```python
from build123d import *

# Parameters (mm, degrees)
SKETCH1_R           = 43.5
BOSS_EXTRUDE1_DEPTH = 122
EXTRUDE_THIN1_START = 0.5
SKETCH1_4_R         = 30.5
SKETCH1_4_R_2       = 30
EXTRUDE_THIN1_DEPTH = 115.5
BOSS_EXTRUDE2_START = 0.8
SKETCH1_5_R         = 42.5
SKETCH1_5_R_2       = 30
BOSS_EXTRUDE2_DEPTH = 115
BOSS_EXTRUDE3_START = 0.3
SKETCH1_6_R         = 43.5
SKETCH1_6_R_2       = 42.5
BOSS_EXTRUDE3_DEPTH = 117
BOSS_EXTRUDE4_START = 1
BOSS_EXTRUDE4_DEPTH = 1
FILLET1_R           = 0.5
SKETCH4_R           = 5.35
CUT_EXTRUDE3_DEPTH  = 180.543866506
CHAMFER1_SIZE       = 1


with BuildPart() as part:
    # Sketch1 → Boss-Extrude1 (new body)
    with BuildSketch(Plane(origin=(0, 0, 0), x_dir=(0, 0, -1), z_dir=(1, 0, 0))):
        Polygon((-66, -28), (-64.5, -26.5), (-64.5, 36), (-43.5, 36), (-22.5, 56), (22.5, 56), (43.5, 36), (64.5, 36), (64.5, -26.5), (66, -28), (66, -58), (26, -58), (24.5, -56.5), (-24.5, -56.5), (-26, -58), (-66, -58), align=None)
        with Locations(Location((0, 0, 0), (0, 0, 180))):
            Circle(SKETCH1_R, mode=Mode.SUBTRACT)
    extrude(amount=BOSS_EXTRUDE1_DEPTH)



with BuildPart() as body_2:
    # Sketch1_4 → Extrude-Thin1 (new body)
    with BuildSketch(Plane(origin=(0, 0, 0), x_dir=(0, 0, -1), z_dir=(1, 0, 0)).offset(EXTRUDE_THIN1_START)):
        Circle(SKETCH1_4_R)
        Circle(SKETCH1_4_R_2, mode=Mode.SUBTRACT)
    extrude(amount=EXTRUDE_THIN1_DEPTH)

    # Sketch1_5 → Boss-Extrude2 (add)
    with BuildSketch(Plane(origin=(0, 0, 0), x_dir=(0, 0, -1), z_dir=(1, 0, 0)).offset(BOSS_EXTRUDE2_START)):
        Circle(SKETCH1_5_R)
        Circle(SKETCH1_5_R_2, mode=Mode.SUBTRACT)
    extrude(amount=BOSS_EXTRUDE2_DEPTH)


with BuildPart() as part_1:
    add(part.part)

    add(body_2.part)  # Boss-Extrude3 merges body 2
    # Sketch1_6 → Boss-Extrude3 (add)
    with BuildSketch(Plane(origin=(0, 0, 0), x_dir=(0, 0, -1), z_dir=(1, 0, 0)).offset(BOSS_EXTRUDE3_START)):
        with Locations(Location((0, 0, 0), (0, 0, 180))):
            Circle(SKETCH1_6_R)
        Circle(SKETCH1_6_R_2, mode=Mode.SUBTRACT)
    extrude(amount=BOSS_EXTRUDE3_DEPTH)

    # Sketch3 → Boss-Extrude4 (add)
    with BuildSketch(Plane(origin=(117.3, 0, 0), x_dir=(0, 0, -1), z_dir=(1, 0, 0)).offset(BOSS_EXTRUDE4_START)):
        with BuildLine():
            Line((-1.000623377, -42.488218989), (-1.024167456, -43.487941789))
            ThreePointArc((-1.024167456, -43.487941789), (0, 43.5), (1.024167456, -43.487941789))
            Line((1.024167456, -43.487941789), (1.000623377, -42.488218989))
            ThreePointArc((1.000623377, -42.488218989), (1.691854541, -41.50157584), (2.830286494, -41.895578267))
            ThreePointArc((2.830286494, -41.895578267), (4.543509208, -41.80773439), (3.658384287, -40.338243836))
            ThreePointArc((3.658384287, -40.338243836), (0, 40.503798481), (-3.658384287, -40.338243836))
            ThreePointArc((-3.658384287, -40.338243836), (-4.543509208, -41.80773439), (-2.830286494, -41.895578267))
            ThreePointArc((-2.830286494, -41.895578267), (-1.691854541, -41.50157584), (-1.000623377, -42.488218989))
        make_face()
    extrude(amount=BOSS_EXTRUDE4_DEPTH)

    # Fillet1
    fillet1_edges = [part_1.edges().sort_by_distance(p)[0] for p in [
        (122, -27.25, 65.25),
        (122, -43, 66),
        (0, 4.75, 64.5),
        (0, 36, 54),
        (0, 46, 33),
        (0, 56, 0),
        (0, 46, -33),
        (0, 36, -54),
        (0, 4.75, -64.5),
        (0, -27.25, -65.25),
        (0, -43, -66),
        (0, -43, 66),
        (0, -27.25, 65.25),
        (61, -26.5, 64.5),
        (61, 36, 64.5),
        (61, 36, 43.5),
        (61, 56, 22.5),
        (61, 56, -22.5),
        (61, 36, -43.5),
        (61, 36, -64.5),
        (61, -26.5, -64.5),
        (61, -28, -66),
        (61, -28, 66),
        (122, -43, -66),
        (122, -27.25, -65.25),
        (122, 4.75, -64.5),
        (122, 36, -54),
        (122, 46, -33),
        (122, 56, 0),
        (122, 46, 33),
        (122, 36, 54),
        (122, 4.75, 64.5),
    ]]
    fillet(fillet1_edges, radius=FILLET1_R)

    # Sketch4 → Cut-Extrude3 (cut, through all)
    with BuildSketch(Plane.XZ.offset(58)):
        with Locations(Location((16, 54, 0), (0, 0, 270))):
            Circle(SKETCH4_R)
        with Locations(Location((106, 54, 0), (0, 0, 270))):
            Circle(SKETCH4_R)
        with Locations(Location((106, -54, 0), (0, 0, 270))):
            Circle(SKETCH4_R)
        with Locations(Location((16, -54, 0), (0, 0, 270))):
            Circle(SKETCH4_R)
    extrude(amount=-CUT_EXTRUDE3_DEPTH, mode=Mode.SUBTRACT)

    # Chamfer1
    chamfer1_edges = [part_1.edges().sort_by_distance(p)[0] for p in [
        (16, 36, -48.65),
        (106, 36, -48.65),
        (106, 36, 59.35),
        (106, -58, 59.35),
        (16, 36, 59.35),
        (16, -58, 59.35),
    ]]
    chamfer(chamfer1_edges, length=CHAMFER1_SIZE)


solid = part_1.part
```
Source: CAD feature listing. Evaluate the final solid. Frame: model axes, mm. A direction names the side the tool comes from. Give positions to 0.01 mm unless a question says otherwise; leave off trailing zeros. Order: outer loops, then holes, each group sorted by start corner. A loop starts at its lowest first (then second) coordinate and runs counter-clockwise, first axis right, second up. Notation, with made-up numbers: (67.5, 69) -> (77.5, 69) arc R30 cw to (77.5, 100) -> close; hole circle Ø10 at (-39.75, -3). An arc over 180 degrees is marked (long way). Use a Markdown table: item, result.
Q1. Section C-C (y = -47). Return the cut outline in (x, z).
A:
| item | result |
|---|---|
| outline | (0, -65.5) arc R0.5 ccw to (0.5, -66) -> (121.5, -66) arc R0.5 ccw to (122, -65.5) -> (122, 65.5) arc R0.5 ccw to (121.5, 66) -> (0.5, 66) arc R0.5 ccw to (0, 65.5) -> close; hole circle Ø10.7 at (16, -54); hole circle Ø10.7 at (16, 54); hole circle Ø10.7 at (106, -54); hole circle Ø10.7 at (106, 54) |
Q2. Section A-A (x = 44.5). Return the cut outline in (y, z).
A:
| item | result |
|---|---|
| outline | (-58, -66) -> (-28.21, -66) arc R0.5 ccw to (-27.85, -65.85) -> (-26.65, -64.65) arc R0.5 cw to (-26.29, -64.5) -> (35.5, -64.5) arc R0.5 ccw to (36, -64) -> (36, -43.7) arc R0.5 cw to (36.14, -43.36) -> (55.86, -22.64) arc R0.5 ccw to (56, -22.3) -> (56, 22.3) arc R0.5 ccw to (55.86, 22.64) -> (36.14, 43.36) arc R0.5 cw to (36, 43.7) -> (36, 64) arc R0.5 ccw to (35.5, 64.5) -> (-26.29, 64.5) arc R0.5 cw to (-26.65, 64.65) -> (-27.85, 65.85) arc R0.5 ccw to (-28.21, 66) -> (-58, 66) -> (-58, 26) -> (-56.5, 24.5) -> (-56.5, -24.5) -> (-58, -26) -> close; hole circle Ø60 at (0, 0) |
Q3. First-contact query: P1, Ø5, axis at y = 34, z = 24.5, coming from the -X side; P2, Ø12.5, axis at x = 106, z = 54, coming from the -Y side; P3, Ø18.5, axis at x = 31.5, y = 8.5, coming from the +Z side; P4, Ø3, axis at x = 52.5, z = 22.5, coming from the -Y side. Flat tips, straight axial feed; report the tip coordinate or a pass-through.
A:
| item | result |
|---|---|
| P1 | x = 0 |
| P2 | y = -57.9 |
| P3 | z = 64.5 |
| P4 | y = -56.5 |
Q4. Material intervals for line 1 (X direction, y = -17, z = 51); line 2 (Z direction, x = 104.5, y = -31.5); line 3 (Y direction, x = 33, z = 0), sorted ascending. Write a range as [from, to].
A:
| item | result |
|---|---|
| line 1 | [0, 11.57], [20.43, 101.57], [110.43, 122] |
| line 2 | [-66, -59.14], [-48.86, 48.86], [59.14, 66] |
| line 3 | [-56.5, -30], [30, 56] |
Q5. Pull-direction query (Y, two-part tool) for faces 1 (the face through (121.86, 46.03, 32.75)), 2 (the face through (119.3, 36, -20)), 3 (the face through (60, 5, -64.5)); classes: +Y half, -Y half, draft (parallel to the pull), parting line (faces both ways), or undercut.
A:
| item | result |
|---|---|
| face 1 | +Y half |
| face 2 | undercut |
| face 3 | draft |
Q6. Section B-B (z = -54). Return the cut outline in (x, y), and give its area (3 significant figures).
A:
| item | result |
|---|---|
| outline | (0, -58) -> (10.65, -58) -> (10.65, 35) -> (9.65, 36) -> (0.5, 36) arc R0.5 ccw to (0, 35.5) -> close; (21.35, -58) -> (100.65, -58) -> (100.65, 35) -> (99.65, 36) -> (22.35, 36) -> (21.35, 35) -> close; (111.35, -58) -> (122, -58) -> (122, 35.5) arc R0.5 ccw to (121.5, 36) -> (112.35, 36) -> (111.35, 35) -> close |
| area | 9,450 mm^2 |
Q7. Section D-D (y = 0). State how many separate pieces and enclosed holes the cut face has, and give its area (3 significant figures).
A:
| item | result |
|---|---|
| separate pieces | 2 |
| enclosed holes | 4 |
| area | 7,880 mm^2 |
Q8. Access query for faces 4 (the face through (0.8, 29, 10)), 5 (the face through (116.54, -25.861, 33.727)), 6 (the face through (60, -56.5, 0)). Directions: +Z, -Z, +X, -X, +Y, -Y. A direction counts if a zero-diameter tool reaches every point of the face in a straight line with its end or side. Return the directions, or none.
A:
| item | result |
|---|---|
| face 4 | -X |
| face 5 | none |
| face 6 | +X, -X, -Y |
